Read the model definition and answer for the solid it produces. Units are mm, in the model's axes. A direction names the side the tool comes from. Round coordinates to 2 decimals unless told otherwise and drop trailing zeros. Order: outer loops, then holes, each group sorted by start corner. A loop starts at its lowest first (then second) coordinate and runs counter-clockwise, first axis right, second up. Notation, with made-up numbers: (-35.75, 9.5) -> (13.25, 9.5) arc R28 ccw to (13.25, 32.5) -> close; hole circle Ø9 at (37.25, 57.25). An arc over 180 degrees is marked (long way). Answer as a JSON object with one key per item and string values. Group by question number.
Item 1: For faces 5 (the flat face through (0, 7, -1.1)), 6 (the cylindrical face through (7.826, 15.477, -0.892)), 7 (the flat face through (-8, 13, 1.5)), 8 (the flat face through (-1, -1, 2)), determine the directions among +Z, -Z, +X, -X, +Y, -Y from which every point of the face is accessible in a straight line to the end or side of a thin tool.
Item 2: Given P1, Ø1.7, axis at y = 11, z = 6, coming from the -X side; P2, Ø1.7, axis at y = 11, z = 6, coming from the +X side; P3, Ø1.6, axis at y = 12.5, z = -1.5, coming from the +X side; P4, Ø2.5, axis at x = 1.5, y = 4.5, coming from the -Z side, each flat-ended and moving along its own axis, determine where each tip first touches the part or whether it passes through.
Item 3: The mould has two halves that part along Z. Classify faces 1 (the cylindrical face through (-4.72, 5.27, 4.37)), 2 (the flat face through (-7.826, 15.12, 0.144)), 3 (the cylindrical face through (-5.92, 21.75, -1.13)), 4 (the flat face through (6.875, 11, -1)): pulls with the +Z half, pulls with the -Z half, needs draft (parallel to the pull), parting line crosses it, or undercut.
Item 4: Section D-D, the plane x = 7.5 is taken. Write down the section's boundary in (y, z), plus the area to 3 significant figures.
Item 5: Section C-C, the plane z = 6 is taken. Count the separate pieces of the cut face and the enclosed holes in it, plus the area to 3 significant figures.
Item 6: Consider probe 1 along X at (y, z) = (-1.5, 4.5); probe 2 along Y at (x, z) = (-5.35, -1.25); probe 3 along X at (y, z) = (16, 5.25). Determine where each line is inside the solid, lowest interval first. Write a range as from..to.
from build123d import *
from build123d.topology import SkipClean

# Parameters (mm, degrees)
BOSS_EXTRUDE1_DEPTH = 22.5
SKETCH3_W           = 10
SKETCH3_H           = 20
CUT_EXTRUDE1_DEPTH  = 17.5
SKETCH4_OUTSIDE_W   = 28.964
SKETCH4_OUTSIDE_H   = 31.464
SKETCH4_OUTSIDE_R   = 1.6
SKETCH4_OUTSIDE_R_2 = 0.75
CUT_EXTRUDE2_DEPTH  = 31.207614934
FILLET1_R           = 1.875
SKETCH7_W           = 20
SKETCH7_H           = 25
CUT_EXTRUDE4_DEPTH  = 8.75
BOSS_EXTRUDE3_DEPTH = 5
FILLET2_R           = 0.9375
SKETCH11_R          = 2.75
CUT_EXTRUDE6_DEPTH  = 1.875
CUT_EXTRUDE7_DEPTH  = 1.875
BOSS_EXTRUDE4_DEPTH = 0.2
BOSS_EXTRUDE9_START = 2.5
BOSS_EXTRUDE9_DEPTH = 2.5
CUT_EXTRUDE8_DEPTH  = 28.895609137


with BuildPart() as part:
    # Sketch2 → Boss-Extrude1 (new body)
    with BuildSketch(Plane(origin=(0, 0, 0), x_dir=(1, 0, 0), z_dir=(0, 1, 0))):
        Polygon((5, 10), (8.75, 10), (8.75, -10), (-8.75, -10), (-8.75, 10), (-5, 10), (-5, 5), (5, 5), align=None)
    extrude(amount=BOSS_EXTRUDE1_DEPTH)

    # Sketch3 → Cut-Extrude1 (cut)
    with BuildSketch(Plane(origin=(0, 22.5, 0), x_dir=(1, 0, 0), z_dir=(0, 1, 0))):
        Rectangle(SKETCH3_W, SKETCH3_H)
    extrude(amount=-CUT_EXTRUDE1_DEPTH, mode=Mode.SUBTRACT)

    # Sketch4 outside → Cut-Extrude2 (cut, through all)
    # profile 1 of 3: a face of its own
    with BuildSketch(Plane(origin=(8.75, 0, 0), x_dir=(0, 0, -1), z_dir=(1, 0, 0))):
        with Locations((0, 11.25)):
            Rectangle(SKETCH4_OUTSIDE_W, SKETCH4_OUTSIDE_H)
        with BuildLine():
            Line((10, 14.856537443), (10, 0))
            Line((10, 0), (-10, 0))
            Line((-10, 0), (-10, 4.952182367))
            Line((-10, 4.952182367), (-7.476419244, 14.952182367))
            ThreePointArc((-7.476419244, 14.952182367), (1.29925445, 21.749865221), (10, 14.856537443))
        make_face(mode=Mode.SUBTRACT)
    # profile 2 of 3: a face of its own
    with BuildSketch(Plane(origin=(8.75, 0, 0), x_dir=(0, 0, -1), z_dir=(1, 0, 0))):
        with Locations((1.25, 12.75)):
            Circle(SKETCH4_OUTSIDE_R)
    # profile 3 of 3: a face of its own
    with BuildSketch(Plane(origin=(8.75, 0, 0), x_dir=(0, 0, -1), z_dir=(1, 0, 0))):
        with Locations((-6, 11)):
            Circle(SKETCH4_OUTSIDE_R_2)
    extrude(amount=-CUT_EXTRUDE2_DEPTH, mode=Mode.SUBTRACT)

    # Fillet1
    # the kernel refuses this fillet: 1.875 mm, written as the material it takes off along each edge
    with BuildSketch(Plane(origin=(-8.75, -1.875, 10), x_dir=(1, 0, 0), z_dir=(0, 1, 0)), Plane(origin=(8.75, -1.875, 10), x_dir=(0, 0, -1), z_dir=(0, 1, 0))) as fillet1_piece_1:
        with BuildLine():
            CenterArc((FILLET1_R, FILLET1_R), FILLET1_R, 180, 90)
            Line((0, FILLET1_R), (-FILLET1_R * 0.02, FILLET1_R))
            Line((-FILLET1_R * 0.02, FILLET1_R), (-FILLET1_R * 0.02, -FILLET1_R * 0.02))
            Line((-FILLET1_R * 0.02, -FILLET1_R * 0.02), (FILLET1_R, -FILLET1_R * 0.02))
            Line((FILLET1_R, -FILLET1_R * 0.02), (FILLET1_R, 0))
        make_face()
    extrude(amount=8.702182367, mode=Mode.SUBTRACT)
    with BuildSketch(Plane(origin=(-8.75, -1.875, -10), x_dir=(0, 0, 1), z_dir=(0, 1, 0)), Plane(origin=(8.75, -1.875, -10), x_dir=(-1, 0, 0), z_dir=(0, 1, 0))) as fillet1_piece_2:
        with BuildLine():
            CenterArc((FILLET1_R, FILLET1_R), FILLET1_R, 180, 90)
            Line((0, FILLET1_R), (-FILLET1_R * 0.02, FILLET1_R))
            Line((-FILLET1_R * 0.02, FILLET1_R), (-FILLET1_R * 0.02, -FILLET1_R * 0.02))
            Line((-FILLET1_R * 0.02, -FILLET1_R * 0.02), (FILLET1_R, -FILLET1_R * 0.02))
            Line((FILLET1_R, -FILLET1_R * 0.02), (FILLET1_R, 0))
        make_face()
    extrude(amount=18.606537443, mode=Mode.SUBTRACT)
    with BuildSketch(Plane(origin=(8.75, 12.75, -1.25), x_dir=(0, 0.2446869297035112, 0.9696021382156028), z_dir=(0, -0.9696021382156028, 0.2446869297035112))) as fillet1_piece_3:
        with BuildLine():
            CenterArc((9 - FILLET1_R, FILLET1_R), FILLET1_R, 270, 90)
            Line((9, FILLET1_R), (9 + FILLET1_R * 0.02, FILLET1_R))
            Line((9 + FILLET1_R * 0.02, FILLET1_R), (9 + FILLET1_R * 0.02, -FILLET1_R * 0.02))
            Line((9 + FILLET1_R * 0.02, -FILLET1_R * 0.02), (9 - FILLET1_R, -FILLET1_R * 0.02))
            Line((9 - FILLET1_R, -FILLET1_R * 0.02), (9 - FILLET1_R, 0))
        make_face()
    revolve(axis=Axis((8.75, 12.75, -1.25), (-1, 0, 0)), revolution_arc=164.250823416, mode=Mode.SUBTRACT)
    with BuildSketch(Plane(origin=(-8.75, 12.75, -1.25), x_dir=(0, 0.027674657987308005, -0.9996169833017472), z_dir=(0, -0.9996169833017472, -0.027674657987308005))) as fillet1_piece_4:
        with BuildLine():
            CenterArc((9 - FILLET1_R, FILLET1_R), FILLET1_R, 270, 90)
            Line((9, FILLET1_R), (9 + FILLET1_R * 0.02, FILLET1_R))
            Line((9 + FILLET1_R * 0.02, FILLET1_R), (9 + FILLET1_R * 0.02, -FILLET1_R * 0.02))
            Line((9 + FILLET1_R * 0.02, -FILLET1_R * 0.02), (9 - FILLET1_R, -FILLET1_R * 0.02))
            Line((9 - FILLET1_R, -FILLET1_R * 0.02), (9 - FILLET1_R, 0))
        make_face()
    revolve(axis=Axis((-8.75, 12.75, -1.25), (1, 0, 0)), revolution_arc=164.250823416, mode=Mode.SUBTRACT)
    with BuildSketch(Plane(origin=(-8.75, 14.952182367, 7.476419244), x_dir=(0, -0.2446869297035113, -0.9696021382156028), z_dir=(0, -0.9696021382156028, 0.24468692970351133)), Plane(origin=(8.75, 3.134178358, 10.458787993), x_dir=(0, -0.24468692970351133, -0.9696021382156028), z_dir=(0, 0.9696021382156028, -0.24468692970351133))) as fillet1_piece_5:
        with BuildLine():
            CenterArc((FILLET1_R, FILLET1_R), FILLET1_R, 180, 90)
            Line((0, FILLET1_R), (-FILLET1_R * 0.02, FILLET1_R))
            Line((-FILLET1_R * 0.02, FILLET1_R), (-FILLET1_R * 0.02, -FILLET1_R * 0.02))
            Line((-FILLET1_R * 0.02, -FILLET1_R * 0.02), (FILLET1_R, -FILLET1_R * 0.02))
            Line((FILLET1_R, -FILLET1_R * 0.02), (FILLET1_R, 0))
        make_face()
    extrude(amount=12.188508609, mode=Mode.SUBTRACT)

    # Sketch7 → Cut-Extrude4 (cut)
    with BuildSketch(Plane(origin=(8.75, 0, 0), x_dir=(0, 0, -1), z_dir=(1, 0, 0))):
        with Locations((0, 12.5)):
            Rectangle(SKETCH7_W, SKETCH7_H)
    extrude(amount=-CUT_EXTRUDE4_DEPTH, mode=Mode.SUBTRACT)

    # Sketch8 → Boss-Extrude3 (add)
    with BuildSketch(Plane(origin=(-5, 0, 0), x_dir=(0, 0, -1), z_dir=(1, 0, 0))):
        Polygon((5, 5), (5, 8.4), (1.1, 10.25), (1.1, 5), align=None)
    extrude(amount=BOSS_EXTRUDE3_DEPTH)

    # Fillet2
    fillet2_edges = [part.edges().sort_by_distance(p)[0] for p in [
        (-5, 5, 4.443966417),
        (-2.5, 10.25, -1.1),
        (-2.5, 8.4, -5),
        (-2.5, 5, -1.1),
    ]]
    fillet(fillet2_edges, radius=FILLET2_R)

    # Mirror2: part across plane


with BuildPart() as part_1:
    add(part.part)
    add(part.part.mirror(Plane.ZY))

    # Sketch11 → Cut-Extrude6 (cut)
    with BuildSketch(Plane(origin=(8.75, 0, 0), x_dir=(0, 0, -1), z_dir=(1, 0, 0))):
        with Locations((1.25, 12.75)):
            Circle(SKETCH11_R)
    extrude(amount=-CUT_EXTRUDE6_DEPTH, mode=Mode.SUBTRACT)

    # Sketch12 → Cut-Extrude7 (cut)
    with BuildSketch(Plane.ZY.offset(8.75)):
        Polygon((-1.25, 15.925426481), (-4, 14.33771324), (-4, 11.16228676), (-1.25, 9.574573519), (1.5, 11.16228676), (1.5, 14.33771324), align=None)
    extrude(amount=-CUT_EXTRUDE7_DEPTH, mode=Mode.SUBTRACT)

    # Sketch13 → Boss-Extrude4 (add)
    with BuildSketch(Plane.ZY.offset(8.75)):
        with BuildLine():
            Line((-2.16945613, 9.400976563), (2.048930789, 9.400976563))
            Line((2.048930789, 9.400976563), (2.048930789, 8.9188752))
            Line((2.048930789, 8.9188752), (1.331428371, 8.9188752))
            add(Edge.make_bspline(
                [(1.331428371, 8.9188752), (1.259186082, 8.917703873), (1.128695628, 8.915588118), (0.953618084, 8.895075924), (0.820795157, 8.85890692), (0.722620482, 8.801340017), (0.66418865, 8.710271847), (0.629489236, 8.592812055), (0.605081268, 8.443393165), (0.603495672, 8.332064189), (0.602626703, 8.271051495)],
                knots=[0, 0, 0, 0, 1.473035235, 2.660727346, 3.584016889, 4.269332832, 4.922698946, 5.732321762, 6.757222385, 8, 8, 8, 8], degree=3))
            Line((0.602626703, 8.271051495), (0.602626703, 1.161939611))
            add(Edge.make_bspline(
                [(0.602626703, 1.161939611), (0.603806075, 1.097741152), (0.605941327, 0.981509859), (0.626332927, 0.828112382), (0.653959528, 0.708007797), (0.695819757, 0.652674401), (0.713736001, 0.628991621)],
                knots=[0, 0, 0, 0, 1.387279159, 2.511668523, 3.362991788, 4, 4, 4, 4], degree=3))
            add(Edge.make_bspline(
                [(0.713736001, 0.628991621), (0.742216021, 0.605874577), (0.803795028, 0.555891305), (0.927817777, 0.514891851), (1.077003332, 0.485769381), (1.186830669, 0.483395223), (1.246683991, 0.482101362)],
                knots=[0, 0, 0, 0, 0.773484526, 1.672414867, 2.731520698, 4, 4, 4, 4], degree=3))
            Line((1.246683991, 0.482101362), (2.048930789, 0.482101362))
            Line((2.048930789, 0.482101362), (2.048930789, 0))
            Line((2.048930789, 0), (-2.16945613, 0))
            Line((-2.16945613, 0), (-2.16945613, 0.482101362))
            Line((-2.16945613, 0.482101362), (-1.382274999, 0.482101362))
            add(Edge.make_bspline(
                [(-1.382274999, 0.482101362), (-1.31940414, 0.48301697), (-1.204997391, 0.484683112), (-1.050781582, 0.508492708), (-0.931283172, 0.545116887), (-0.839180191, 0.603218278), (-0.785035731, 0.698739607), (-0.746995159, 0.820804221), (-0.726559461, 0.979920139), (-0.7243631, 1.097246659), (-0.723152043, 1.161939611)],
                knots=[0, 0, 0, 0, 1.323224596, 2.407885381, 3.273374914, 3.948198526, 4.637756618, 5.528332226, 6.637141158, 8, 8, 8, 8], degree=3))
            Line((-0.723152043, 1.161939611), (-0.723152043, 8.271051495))
            add(Edge.make_bspline(
                [(-0.723152043, 8.271051495), (-0.724696232, 8.332673526), (-0.727462884, 8.443078849), (-0.743603421, 8.589300261), (-0.77489184, 8.700371502), (-0.815344506, 8.750765334), (-0.832378133, 8.771984942)],
                knots=[0, 0, 0, 0, 1.411879347, 2.529598496, 3.380849948, 4, 4, 4, 4], degree=3))
            add(Edge.make_bspline(
                [(-0.832378133, 8.771984942), (-0.866044035, 8.795002172), (-0.940377737, 8.845823799), (-1.084531483, 8.88950754), (-1.261441827, 8.914084364), (-1.390944762, 8.917187619), (-1.461369754, 8.9188752)],
                knots=[0, 0, 0, 0, 0.741247183, 1.636660366, 2.714792252, 4, 4, 4, 4], degree=3))
            Line((-1.461369754, 8.9188752), (-2.16945613, 8.9188752))
            Line((-2.16945613, 8.9188752), (-2.16945613, 9.400976563))
        make_face()
    extrude(amount=BOSS_EXTRUDE4_DEPTH)

    # Sketch19 → Boss-Extrude9 (add)
    with SkipClean():  # the faces are left unmerged after this step: merging them gives an invalid solid
        with BuildSketch(Plane.XZ.offset(BOSS_EXTRUDE9_START)):
            with BuildLine():
                Line((-8.75, 2.048930789), (-8.75, -2.16945613))
                Line((-8.75, -2.16945613), (-8.75, -8.125))
                ThreePointArc((-8.75, -8.125), (-8.200825215, -9.450825215), (-6.875, -10))
                Line((-6.875, -10), (-5, -10))
                Line((-5, -10), (-5, -5))
                Line((-5, -5), (5, -5))
                Line((5, -5), (5, -10))
                Line((5, -10), (6.875, -10))
                ThreePointArc((6.875, -10), (8.200825215, -9.450825215), (8.75, -8.125))
                Line((8.75, -8.125), (8.75, 8.125))
                ThreePointArc((8.75, 8.125), (8.200825215, 9.450825215), (6.875, 10))
                Line((6.875, 10), (-6.875, 10))
                ThreePointArc((-6.875, 10), (-8.200825215, 9.450825215), (-8.75, 8.125))
                Line((-8.75, 8.125), (-8.75, 2.048930789))
            make_face()
        extrude(amount=-BOSS_EXTRUDE9_DEPTH)

    # Sketch20 → Cut-Extrude8 (cut, through all)
    with SkipClean():  # the faces are left unmerged after this step: merging them gives an invalid solid
        with BuildSketch(Plane(origin=(0, 0, -5), x_dir=(-1, 0, 0), z_dir=(0, 0, -1))):
            with BuildLine():
                Line((1, 0.25), (2.5, 0.25))
                ThreePointArc((2.5, 0.25), (3.5, 1.25), (2.5, 2.25))
                Line((2.5, 2.25), (-2.5, 2.25))
                ThreePointArc((-2.5, 2.25), (-3.5, 1.25), (-2.5, 0.25))
                Line((-2.5, 0.25), (-1, 0.25))
                Line((-1, 0.25), (-1, -2.5))
                ThreePointArc((-1, -2.5), (0, -3.5), (1, -2.5))
                Line((1, -2.5), (1, 0.25))
            make_face()
        extrude(amount=-CUT_EXTRUDE8_DEPTH, mode=Mode.SUBTRACT)


solid = part_1.part
Values found:
{
 "1": {"face 5": "+Z, +Y", "face 6": "+X", "face 7": "-X", "face 8": "+Z, -Z, -Y"},
 "2": {"P1": "x = -8.75", "P2": "x = 8.75", "P3": "through", "P4": "z = -5"},
 "3": {"face 1": "needs draft", "face 2": "undercut", "face 3": "parting line crosses it", "face 4": "undercut"},
 "4": {"outline": "(-2.5, -9.89) -> (14.84, -9.89) arc R8.89 ccw to (14.93, 7.37) -> (4.94, 9.89) -> (-2.5, 9.89) -> close; hole circle Ø5.5 at (12.75, -1.25); hole circle Ø1.5 at (11, 6)", "area": "393 mm2"},
 "5": {"separate pieces": "3", "enclosed holes": "0", "area": "197 mm2"},
 "6": {"probe 1": "-8.75..-1, 1..8.75", "probe 2": "-2.5..11.15, 14.35..21.75", "probe 3": "-8.74..-5, 5..8.74"}
}
